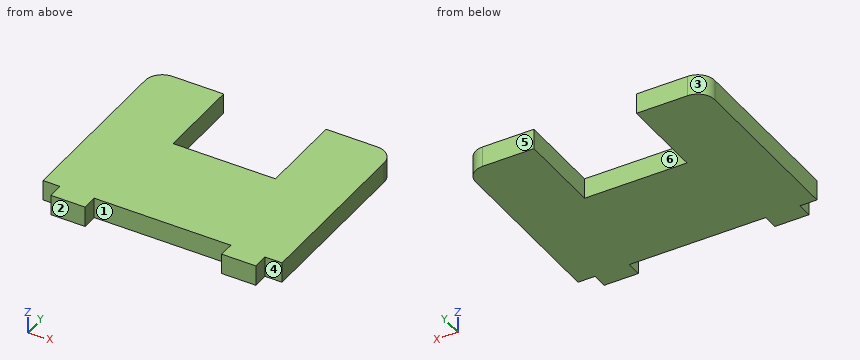
from build123d import *

# Parameters (mm, degrees)
F1_DEPTH = 6


with BuildPart() as f1:
    # F0 (on Top) → F1 (new body)
    with BuildSketch(Plane.XY):
        with BuildLine():
            Line((-35, 20), (-35, -30.5))
            Line((-35, -30.5), (-30, -30.5))
            Line((-30, -30.5), (-30, -35))
            Line((-30, -35), (-20, -35))
            Line((-20, -35), (-20, -30.5))
            Line((-20, -30.5), (20, -30.5))
            Line((20, -30.5), (20, -35))
            Line((20, -35), (30, -35))
            Line((30, -35), (30, -30.5))
            Line((30, -30.5), (35, -30.5))
            Line((35, -30.5), (35, 20))
            ThreePointArc((35, 20), (33.535534, 23.535534), (30, 25))
            Line((30, 25), (15, 25))
            Line((15, 25), (15, 0))
            Line((15, 0), (-15, 0))
            Line((-15, 0), (-15, 25))
            Line((-15, 25), (-30, 25))
            ThreePointArc((-30, 25), (-33.535534, 23.535534), (-35, 20))
        make_face()
    extrude(amount=F1_DEPTH)


solid = f1.part
Design review of the part built by this model. Coordinates are the model's own, in mm. Face numbers are marked on the shaded views. A direction names the side the tool comes from. Coordinates: 2 decimals unless noted, no trailing zeros. Loops run counter-clockwise (first coordinate to the right, second up) from the corner with the lowest first, then second, coordinate; pieces in that order, holes last. Notation, with made-up numbers: (15, -13) -> (45, -13) arc R21 ccw to (45, 6) -> close; hole circle Ø1 at (84.5, 80). An arc over 180 degrees is marked (long way). Use a Markdown table: item, result. Add a question column.
Item 1: Wall thickness on L1, parallel to X at y = -32, z = 2.25; L2, parallel to Y at x = 10.5, z = 0.5; L3, parallel to Y at x = -18, z = 0.35: over which ranges is each line inside the solid? List them lowest first. Write a range as from..to.
Item 2: The part is to be moulded in two halves that separate along X. For the marked faces 1, 2 and 3, say which applies: +X half, -X half, draft (parallel to the pull), parting line (faces both ways), or undercut.
Item 3: We need section A-A, the plane z = 1.55. Write out the cut boundary in (x, y), and give its area (3 significant figures).
Item 4: Clearance check with flat-ended pins moving along their axes: P1, Ø3, axis at x = -0.5, z = 2, coming from the -Y side; P2, Ø1.5, axis at x = -6.5, z = 4.5, coming from the +Y side; P3, Ø1.3, axis at y = -33.5, z = 4, coming from the -X side. State where each tip first meets the part, or that it passes through.
Item 5: Machinability: for the marked faces 4, 5 and 6, which of the approach directions +Z, -Z, +X, -X, +Y, -Y give a long, thin tool a straight path to every point of the face, cutting with its end or side? Answer none if there is none.
Item 6: We need section C-C, the plane x = -17. Write out the cut boundary in (y, z), and give its area (3 significant figures).
Item 7: We need section B-B, the plane x = -7. Write out the cut boundary in (y, z).
Numbers:
| question | item | result |
|---|---|---|
| 1 | L1 | x = -30..-20, 20..30 |
| 1 | L2 | y = -30.5..0 |
| 1 | L3 | y = -30.5..25 |
| 2 | face 1 | undercut |
| 2 | face 2 | draft |
| 2 | face 3 | -X half |
| 3 | outline | (-35, -30.5) -> (-30, -30.5) -> (-30, -35) -> (-20, -35) -> (-20, -30.5) -> (20, -30.5) -> (20, -35) -> (30, -35) -> (30, -30.5) -> (35, -30.5) -> (35, 20) arc R5 ccw to (30, 25) -> (15, 25) -> (15, 0) -> (-15, 0) -> (-15, 25) -> (-30, 25) arc R5 ccw to (-35, 20) -> close |
| 3 | area | 3,210 mm^2 |
| 4 | P1 | stops at y = -30.5 |
| 4 | P2 | stops at y = 0 |
| 4 | P3 | stops at x = -30 |
| 5 | face 4 | +Z, -Z, +X, -Y |
| 5 | face 5 | +Z, -Z, +X, -X, +Y |
| 5 | face 6 | +Z, -Z, +Y |
| 6 | outline | (-30.5, 0) -> (25, 0) -> (25, 6) -> (-30.5, 6) -> close |
| 6 | area | 333 mm^2 |
| 7 | outline | (-30.5, 0) -> (0, 0) -> (0, 6) -> (-30.5, 6) -> close |
